Design review of the part shown in the three views and the two pictorial views. Dimensions are in mm from the part's minimum x, y and z. A direction names the side the tool comes from. Give positions to 0.01 mm unless a question says otherwise; leave off trailing zeros. Order: outer loops, then holes, each group sorted by start corner. A loop starts at its lowest first (then second) coordinate and runs counter-clockwise, first axis right, second up.
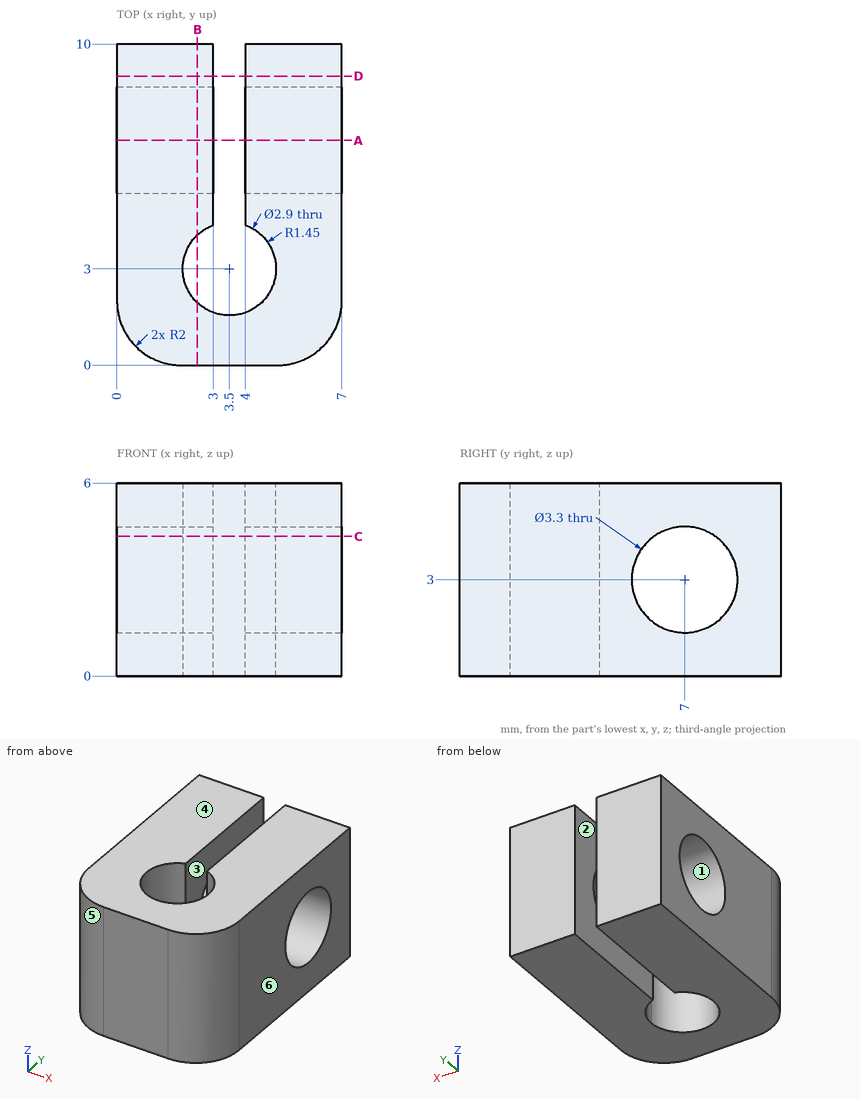
Item 1: Take a section at D-D (y = 9). Give the boundary of the cut face in (x, z), and give its area (3 significant figures).
Values found:
outline: (0, 0) - (3, 0) - (3, 6) - (0, 6) - close; (4, 0) - (7, 0) - (7, 6) - (4, 6) - close
area: 36.0 mm2
Item 2: Take a section at A-A (y = 7). Give the boundary of the cut face in (x, z), and give its area (3 significant figures).
Values found:
outline: (0, 0) - (3, 0) - (3, 1.35) - (0, 1.35) - close; (0, 4.65) - (3, 4.65) - (3, 6) - (0, 6) - close; (4, 0) - (7, 0) - (7, 1.35) - (4, 1.35) - close; (4, 4.65) - (7, 4.65) - (7, 6) - (4, 6) - close
area: 16.2 mm2
Item 3: Take a section at B-B (x = 2.5). Give the boundary of the cut face in (y, z), and give its area (3 significant figures).
Values found:
outline: (0, 0) - (1.95, 0) - (1.95, 6) - (0, 6) - close; (4.05, 0) - (10, 0) - (10, 6) - (4.05, 6) - close; hole circle Ø3.3 at (7, 3)
area: 38.8 mm2
Item 4: Draft analysis for pull direction X (two halves, no side actions). For the marked faces 3, 4, 5 and 6, state which applies: released by +X, released by -X, zero draft, split by the parting line, or undercut.
Values found:
face 3: undercut
face 4: zero draft
face 5: released by -X
face 6: released by +X
Item 5: Take a section at C-C (z = 4.35). Give the boundary of the cut face in (x, y), and give its area (3 significant figures).
Values found:
outline: (0, 2) arc R2 ccw to (2, 0) - (5, 0) arc R2 ccw to (7, 2) - (7, 6.05) - (4, 6.05) - (4, 4.36) arc R1.45 cw (long way) to (3, 4.36) - (3, 6.05) - (0, 6.05) - close; (0, 7.95) - (3, 7.95) - (3, 10) - (0, 10) - close; (4, 7.95) - (7, 7.95) - (7, 10) - (4, 10) - close
area: 44.7 mm2
Item 6: For line 1 (X direction, y = 9.5, z = 0.3); line 2 (Z direction, x = 5.6, y = 7); line 3 (X direction, y = 1.75, z = 2.2), list the stretches that pass through material, from the lowest coordinate up.
Values found:
line 1: x = 0 to 3, 4 to 7
line 2: z = 0 to 1.35, 4.65 to 6
line 3: x = 0.02 to 2.77, 4.23 to 6.98
Item 7: For the marked faces 1 and 2, list the 3-axis set-ups (+Z, -Z, +X, -X, +Y, -Y) from which the entire face can be reached by the end or side of a thin tool; tool diameter is ignored.
Values found:
face 1: +X, -X
face 2: +Z, -Z, +Y
